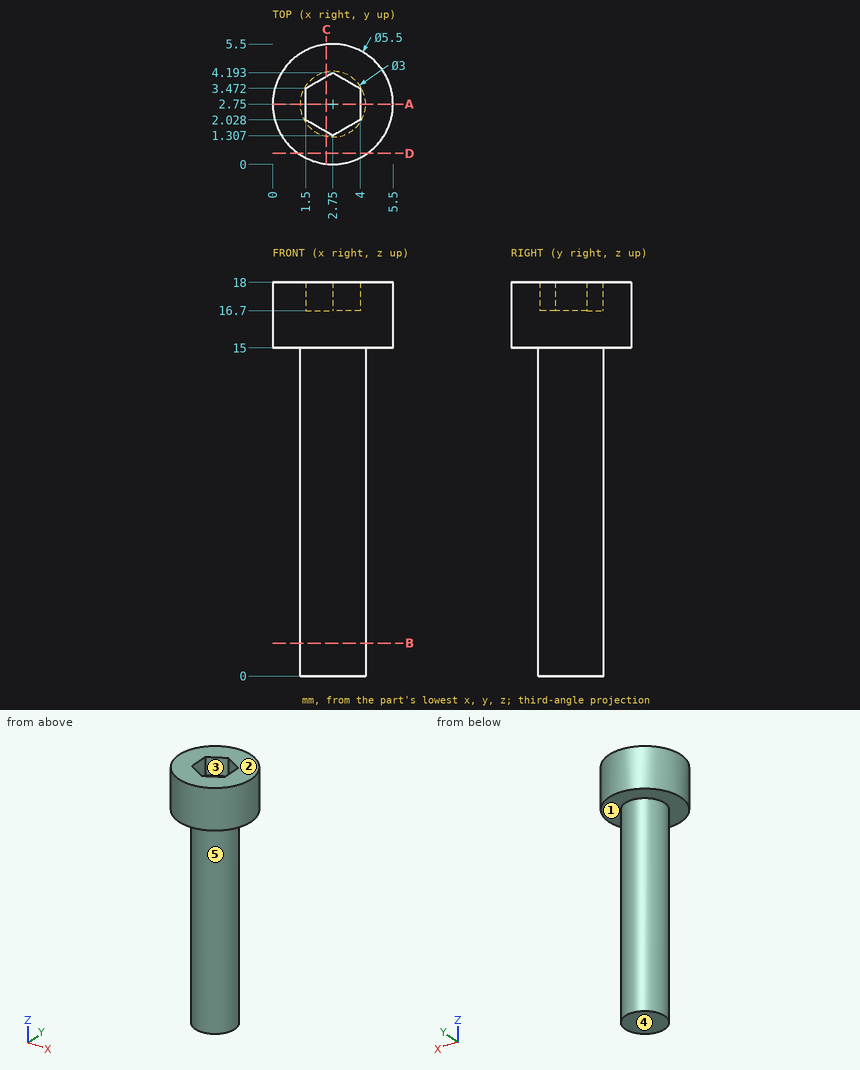
The figure shows three views and two pictorial views of one solid part (mm, origin at its lowest corner). Answer the questions. A direction names the side the tool comes from. Coordinates: 2 decimals unless noted, no trailing zeros. Write each loop counter-clockwise with the first axis right and the second up, starting at its lowest first coordinate (ties: lowest second). Pieces come first, ordered by that corner, then holes. Notation, with made-up numbers: M -12.75,4 L 37.25,4 A31 ccw 37.25,37 Z; hole C 9,47.5 d10. An arc over 180 degrees is marked long. Answer as CSV lines item,"result". Start each with the question number.
Item 1: Determine the mould class of the marked faces 3, 4 and 5 for opening direction X: released by +X, released by -X, zero draft, split by the parting line, or undercut.
Item 2: Flat-ended cylindrical pins translate along their axes: P1, Ø1, axis at y = 2.5, z = 17.5, coming from the +X side; P2, Ø3, axis at x = 0.5, z = 15.5, coming from the +Y side (1 decimal); P3, Ø3, axis at x = 3, z = 6.5, coming from the -Y side. Find the tip coordinate at first contact, or state that the pin passes through.
Item 3: Section C-C on x = 2.45 is taken. Write down the section's boundary in (y, z).
Item 4: Consider L1, parallel to Z at x = 1.5, y = 1.2; L2, parallel to Z at x = 2.05, y = 3.65; L3, parallel to Y at x = 1.95, z = 17.25. Determine where each line is inside the solid, lowest interval first.
Item 5: Section A-A on y = 2.75 is taken. Write down the section's boundary in (x, z).
Item 6: A tool of negligible diameter and unlimited length cuts with its end or side. For the marked faces 1 and 2, from which of +Z, -Z, +X, -X, +Y, -Y can it reach the whole face along a straight path? Write none if from no direction.
Item 7: Section B-B on z = 1.5 is taken. Write down the section's boundary in (x, y).
Item 8: Section D-D on y = 0.5 is taken. Write down the section's boundary in (x, z).
Checks:
1,face 3,"undercut"
1,face 4,"zero draft"
1,face 5,"split by the parting line"
2,P1,"stops at x = 5.5"
2,P2,"stops at y = 5.4"
2,P3,"stops at y = 1.25"
3,outline,"M 0.02,15 L 1.28,15 L 1.28,0 L 4.22,0 L 4.22,15 L 5.48,15 L 5.48,18 L 4.02,18 L 4.02,16.7 L 1.48,16.7 L 1.48,18 L 0.02,18 Z"
4,L1,"z = 15 to 18"
4,L2,"z = 0 to 16.7"
4,L3,"y = 0.12 to 1.77, 3.73 to 5.38"
5,outline,"M 0,15 L 1.25,15 L 1.25,0 L 4.25,0 L 4.25,15 L 5.5,15 L 5.5,18 L 4,18 L 4,16.7 L 1.5,16.7 L 1.5,18 L 0,18 Z"
6,face 1,"-Z"
6,face 2,"+Z, +X, -X, +Y, -Y"
7,outline,"C 2.75,2.75 d3"
8,outline,"M 1.17,15 L 4.33,15 L 4.33,18 L 1.17,18 Z"
